The model under review builds one solid part; all positions refer to its coordinate system, in mm. A direction names the side the tool comes from. Coordinates: 2 decimals unless noted, no trailing zeros. Write each loop counter-clockwise with the first axis right and the second up, starting at its lowest first coordinate (ties: lowest second). Pieces come first, ordered by that corner, then holes.
1) Machinability: for faces 4 (the flat face through (13, 63, -11)), 5 (the flat face through (6, 13, -34)), 6 (the flat face through (-13, 78, -19)), 7 (the flat face through (-19, 80, 0)), 8 (the flat face through (0, 18, 5)), which of the approach directions +Z, -Z, +X, -X, +Y, -Y give a long, thin tool a straight path to every point of the face, cutting with its end or side? Answer none if there is none.
2) Add section C-C, the plane x = -23.5. State the section outline as (y, z) points, then the cut area to 3 significant figures.
3) Mouldability with a two-part tool opening along Y and no side actions: class faces 1 (the flat face through (0, 18, -5)), 2 (the cylindrical face through (10.319, 6.591, 50.466)), 3 (the flat face through (-1, 0, -1)) as released by +Y, released by -Y, zero draft, split by the parting line, or undercut.
4) Add section D-D, the plane z = 7.5. State the section outline as (x, y) points, then the cut area to 3 significant figures.
5) Add section B-B, the plane y = 51. State the section outline as (x, z) points, then the cut area to 3 significant figures.
6) Add section A-A, the plane x = 9.5. State the section outline as (y, z) points.
7) For P1, Ø8, axis at x = -13, y = 83, coming from the +Z side; P2, Ø8, axis at x = -4, y = 32.5, coming from the +Z side; P3, Ø17.5, axis at y = 49, z = -23.5, coming from the +X side; P4, Ø11, axis at x = 13, z = -44, coming from the -Y side, all flat-tipped, find the tip position at first contact; note any pin that passes through.
8) For line 1 (X direction, y = 8.75, z = -44); line 2 (Y direction, x = 9, z = 10); line 3 (Z direction, x = 6.5, y = 22.5), list the stretches that pass through material, from the lowest coordinate up.
from build123d import *

# Parameters (mm, degrees)
SKETCH1_W           = 76
SKETCH1_H           = 126
BOSS_EXTRUDE1_DEPTH = 13
SKETCH2_W           = 13
SKETCH2_H           = 126
BOSS_EXTRUDE2_DEPTH = 77
FILLET1_R           = 25
SKETCH3_W           = 18
SKETCH3_H           = 10
CUT_EXTRUDE1_DEPTH  = 127.641225515
BOSS_EXTRUDE3_DEPTH = 25
SKETCH3_4_R         = 25
SKETCH3_4_R_2       = 16
BOSS_EXTRUDE4_DEPTH = 38
RIB1_REACH          = 118.245
SKETCH4_WALL_W      = 262.668865642
SKETCH4_WALL_H      = 10
SKETCH5_R           = 7
CUT_EXTRUDE2_DEPTH  = 107.498826285
SKETCH3_5_R         = 16
CUT_EXTRUDE3_DEPTH  = 127.641225515


with BuildPart() as part:
    # Sketch1 → Boss-Extrude1 (new body)
    with BuildSketch(Plane(origin=(0, 0, 0), x_dir=(1, 0, 0), z_dir=(0, 1, 0))):
        Rectangle(SKETCH1_W, SKETCH1_H)
    extrude(amount=BOSS_EXTRUDE1_DEPTH)

    # Sketch2 → Boss-Extrude2 (add)
    with BuildSketch(Plane(origin=(0, 13, 0), x_dir=(1, 0, 0), z_dir=(0, 1, 0))):
        with Locations((-31.5, 0)):
            Rectangle(SKETCH2_W, SKETCH2_H)
    extrude(amount=BOSS_EXTRUDE2_DEPTH)

    # Fillet1
    fillet1_edges = [part.edges().sort_by_distance(p)[0] for p in [
        (-31.5, 90, 63),
        (-31.5, 90, -63),
    ]]
    fillet(fillet1_edges, radius=FILLET1_R)

    # Sketch3 → Cut-Extrude1 (cut, through all)
    with BuildSketch(Plane(origin=(-25, 0, 0), x_dir=(0, 0, -1), z_dir=(1, 0, 0))):
        with Locations((0, 85)):
            Rectangle(SKETCH3_W, SKETCH3_H)
    extrude(amount=-CUT_EXTRUDE1_DEPTH, mode=Mode.SUBTRACT)

    # Sketch3_3 → Boss-Extrude3 (add)
    with BuildSketch(Plane(origin=(-25, 0, 0), x_dir=(0, 0, -1), z_dir=(1, 0, 0))):
        with BuildLine():
            Line((-9, 80), (-9, 90))
            Line((-9, 90), (-19, 90))
            Line((-19, 90), (-19, 67.248076809))
            ThreePointArc((-19, 67.248076809), (0, 76), (19, 67.248076809))
            Line((19, 67.248076809), (19, 90))
            Line((19, 90), (9, 90))
            Line((9, 90), (9, 80))
            Line((9, 80), (-9, 80))
        make_face()
    extrude(amount=BOSS_EXTRUDE3_DEPTH)

    # Sketch3_4 → Boss-Extrude4 (add)
    with BuildSketch(Plane(origin=(-25, 0, 0), x_dir=(0, 0, -1), z_dir=(1, 0, 0))):
        with Locations(Location((0, 51, 0), (0, 0, 139.464197889))):
            Circle(SKETCH3_4_R)
        with Locations((0, 51)):
            Circle(SKETCH3_4_R_2, mode=Mode.SUBTRACT)
    extrude(amount=BOSS_EXTRUDE4_DEPTH)

    # Sketch4 wall → Rib1 (add, up to next)
    with BuildSketch(Plane(origin=(25.5, 19.5, 0), x_dir=(0.887216801235, -0.461352736642, 0), z_dir=(0.461352736642, 0.887216801235, 0)), mode=Mode.PRIVATE) as rib1_sk1:
        Rectangle(SKETCH4_WALL_W, SKETCH4_WALL_H)
    rib1_tool1 = extrude(rib1_sk1.sketch, amount=-RIB1_REACH, mode=Mode.PRIVATE) - part.part
    add(rib1_tool1.solids().sort_by_distance((25.5, 19.5, 0))[0])

    # Sketch5 → Cut-Extrude2 (cut, through all)
    with BuildSketch(Plane(origin=(0, 13, 0), x_dir=(1, 0, 0), z_dir=(0, 1, 0))):
        with Locations(Location((13, -44, 0), (0, 0, 270))):
            Circle(SKETCH5_R)
        with Locations(Location((13, 44, 0), (0, 0, 270))):
            Circle(SKETCH5_R)
    extrude(amount=-CUT_EXTRUDE2_DEPTH, mode=Mode.SUBTRACT)

    # Sketch3_5 → Cut-Extrude3 (cut, through all)
    with BuildSketch(Plane(origin=(-25, 0, 0), x_dir=(0, 0, -1), z_dir=(1, 0, 0))):
        with Locations((0, 51)):
            Circle(SKETCH3_5_R)
    extrude(amount=-CUT_EXTRUDE3_DEPTH, mode=Mode.SUBTRACT)


solid = part.part
Geometry results:
1. face 4: +Z, -Z, +X, +Y
1. face 5: -Z, +X
1. face 6: -Z, +X, +Y
1. face 7: +X, -X, +Y
1. face 8: +Z, +X
2. outline: (0, -63) - (13, -63) - (13, -5) - (26.51, -5) arc R25 ccw to (67.25, -19) - (90, -19) - (90, -9) - (80, -9) - (80, 9) - (90, 9) - (90, 19) - (67.25, 19) arc R25 ccw to (26.51, 5) - (13, 5) - (13, 63) - (0, 63) - close; hole circle Ø32 at (51, 0)
2. area: 3,380 mm2
3. face 1: undercut
3. face 2: zero draft
3. face 3: released by -Y
4. outline: (-38, 0) - (38, 0) - (38, 13) - (-25, 13) - (-25, 27.15) - (13, 27.15) - (13, 36.87) - (-38, 36.87) - close; (-38, 65.13) - (13, 65.13) - (13, 74.85) - (0, 74.85) - (0, 80) - (-38, 80) - close
4. area: 2,360 mm2
5. outline: (-38, -63) - (-25, -63) - (-25, -25) - (13, -25) - (13, -16) - (-38, -16) - close; (-38, 16) - (13, 16) - (13, 25) - (-25, 25) - (-25, 63) - (-38, 63) - close
5. area: 1,910 mm2
6. outline: (0, -63) - (13, -63) - (13, -50.06) - (0, -50.06) - close; (0, -37.94) - (13, -37.94) - (13, -5) - (26.51, -5) arc R25 ccw (long way) to (26.51, 5) - (13, 5) - (13, 37.94) - (0, 37.94) - close; (0, 50.06) - (13, 50.06) - (13, 63) - (0, 63) - close; hole circle Ø32 at (51, 0)
7. P1: stops at z = 19
7. P2: stops at z = 20.37
7. P3: stops at x = 13
7. P4: passes through
8. line 1: x = -38 to 6, 20 to 38
8. line 2: y = 0 to 13, 28.09 to 38.51, 63.49 to 73.91
8. line 3: z = -5 to 5
